Work out the finished part from the listing and answer in its coordinate system (mm). A direction names the side the tool comes from. Round coordinates to 2 decimals unless told otherwise and drop trailing zeros. Order: outer loops, then holes, each group sorted by start corner. A loop starts at its lowest first (then second) coordinate and runs counter-clockwise, first axis right, second up. Notation, with made-up numbers: (36.5, 67.25) - (61.5, 67.25) arc R6 ccw to (61.5, 71.25) - close; hole circle Ø10 at (15.25, 69). An arc over 180 degrees is marked (long way). Answer in a Markdown table with one row per item.
from build123d import *

# Parameters (mm, degrees)
SKETCH_1_R          = 1.9
EXTRUDE_1_DEPTH     = 1.4
CUT_EXTRUDE_1_DEPTH = 1
FILLET_1_R          = 1
SKETCH_3_R          = 0.95
EXTRUDE_2_DEPTH     = 8
CHAMFER_1_SIZE      = 0.2


with BuildPart() as part:
    # 草图1 → 凸台-拉伸1 (new body)
    with BuildSketch(Plane(origin=(0, 0, 0), x_dir=(1, 0, 0), z_dir=(0, 1, 0))):
        Circle(SKETCH_1_R)
    extrude(amount=EXTRUDE_1_DEPTH)

    # 草图2 → 切除-拉伸1 (cut)
    with BuildSketch(Plane(origin=(0, 1.4, 0), x_dir=(1, 0, 0), z_dir=(0, 1, 0))):
        Polygon((0, -0.866025404), (0.75, -0.433012702), (0.75, 0.433012702), (0, 0.866025404), (-0.75, 0.433012702), (-0.75, -0.433012702), align=None)
    extrude(amount=-CUT_EXTRUDE_1_DEPTH, mode=Mode.SUBTRACT)

    # 圆角1
    fillet_1_edges = [part.edges().sort_by_distance(p)[0] for p in [
        (-1.9, 1.4, 0),
    ]]
    fillet(fillet_1_edges, radius=FILLET_1_R)

    # 草图3 → 凸台-拉伸2 (add)
    with BuildSketch(Plane.XZ):
        Circle(SKETCH_3_R)
    extrude(amount=EXTRUDE_2_DEPTH)

    # 倒角1
    chamfer_1_edges = [part.edges().sort_by_distance(p)[0] for p in [
        (-0.95, -8, 0),
    ]]
    chamfer(chamfer_1_edges, length=CHAMFER_1_SIZE)


solid = part.part
1) Which of the six approach directions +Z, -Z, +X, -X, +Y, -Y give full straight-line access (tool end or side, diameter ignored) to faces 1 (the face through (-1.9, 0.2, -0.08)), 2 (the face through (0.75, 1, 0))?
Filled in:
| item | result |
|---|---|
| face 1 | +Y, -Y |
| face 2 | +Y |
2) The mould has two halves that part along Z. Classify faces 3 (the face through (-0.95, -3.85, 0.04)), 4 (the face through (-0.75, 1, 0)), 5 (the face through (0, 0.4, 0)), 6 (the face through (1, 0, 1)): released by +Z, released by -Z, zero draft, split by the parting line, or undercut.
Filled in:
| item | result |
|---|---|
| face 3 | split by the parting line |
| face 4 | undercut |
| face 5 | undercut |
| face 6 | zero draft |
3) Find the intervals of material crossed by probe 1 along X at (y, z) = (-6.5, 0.3); probe 2 along Z at (x, y) = (0.2, 0.5); probe 3 along Y at (x, z) = (-1.45, 1.05), in increasing order. Write a range as from..to.
Filled in:
| item | result |
|---|---|
| probe 1 | x = -0.9..0.9 |
| probe 2 | z = -1.88..-0.75, 0.75..1.88 |
| probe 3 | y = 0..0.86 |
4) Find section A-A, the plane y = -6.25. Give the vertices of the cut face in (x, z).
Filled in:
| item | result |
|---|---|
| outline | circle Ø1.9 at (0, 0) |
5) Each of these flat-tipped pins is pushed along its axis until it touches: pin 1 (0.8 mm diameter, centred on x = 0, z = 0, fed in from +Y); pin 2 (2 mm diameter, centred on x = -1, y = -5.5, fed in from -Z); pin 3 (1.5 mm diameter, centred on x = -1.5, z = -0.5, fed in from -Y). Where does it stop, or does it pass through?
Filled in:
| item | result |
|---|---|
| pin 1 | stops at y = 0.4 |
| pin 2 | stops at z = -0.95 |
| pin 3 | stops at y = -7.92 |
